```python
from build123d import *

# Parameters (mm, degrees)
SKETCH1_W           = 30
SKETCH1_H           = 44
BOSS_EXTRUDE2_DEPTH = 1


with BuildPart() as part:
    # Sketch1 → Boss-Extrude2 (new body)
    with BuildSketch(Plane.XY):
        Rectangle(SKETCH1_W, SKETCH1_H)
        with BuildLine():
            Line((-7, 8), (7, 8))
            ThreePointArc((7, 8), (7.707106781, 8.292893219), (8, 9))
            Line((8, 9), (8, 12))
            ThreePointArc((8, 12), (7.707106781, 12.707106781), (7, 13))
            Line((7, 13), (-7, 13))
            ThreePointArc((-7, 13), (-7.707106781, 12.707106781), (-8, 12))
            Line((-8, 12), (-8, 9))
            ThreePointArc((-8, 9), (-7.707106781, 8.292893219), (-7, 8))
        make_face(mode=Mode.SUBTRACT)
        with BuildLine():
            Line((-7, -4), (7, -4))
            ThreePointArc((7, -4), (7.707106781, -3.707106781), (8, -3))
            Line((8, -3), (8, 3))
            ThreePointArc((8, 3), (7.707106781, 3.707106781), (7, 4))
            Line((7, 4), (-7, 4))
            ThreePointArc((-7, 4), (-7.707106781, 3.707106781), (-8, 3))
            Line((-8, 3), (-8, -3))
            ThreePointArc((-8, -3), (-7.707106781, -3.707106781), (-7, -4))
        make_face(mode=Mode.SUBTRACT)
        with BuildLine():
            Line((-7, -13), (7, -13))
            ThreePointArc((7, -13), (7.707106781, -12.707106781), (8, -12))
            Line((8, -12), (8, -9))
            ThreePointArc((8, -9), (7.707106781, -8.292893219), (7, -8))
            Line((7, -8), (-7, -8))
            ThreePointArc((-7, -8), (-7.707106781, -8.292893219), (-8, -9))
            Line((-8, -9), (-8, -12))
            ThreePointArc((-8, -12), (-7.707106781, -12.707106781), (-7, -13))
        make_face(mode=Mode.SUBTRACT)
    extrude(amount=BOSS_EXTRUDE2_DEPTH)


solid = part.part
```
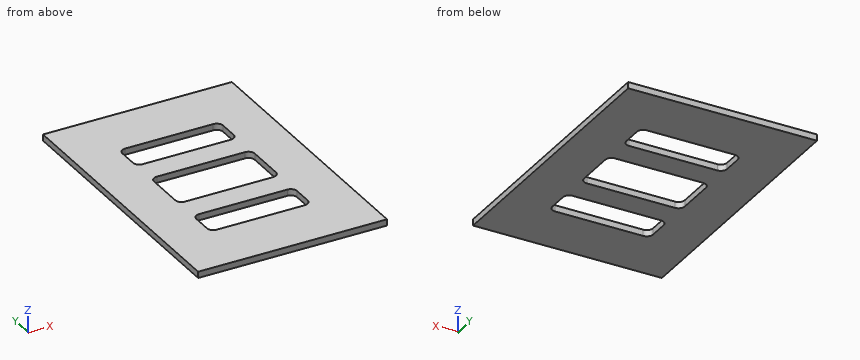
Input: part model. Units: mm. Frame: model coordinates. Coordinates: 2 decimals unless noted, no trailing zeros. Loops run counter-clockwise (first coordinate to the right, second up) from the corner with the lowest first, then second, coordinate; pieces in that order, holes last. Notation, with made-up numbers: M 53,-25 L 82,-25 A27 ccw 82,-7 Z; hole C 19.25,14.25 d8. An arc over 180 degrees is marked long. One line per item, written item: value.
(1) Section A-A (y = 2). Output: boundary loops of the cut face in (x, z).
Filled in:
outline: M -15,0 L -8,0 L -8,1 L -15,1 Z; M 8,0 L 15,0 L 15,1 L 8,1 Z
(2) Section C-C (z = 0.45). Output: boundary loops of the cut face in (x, y).
Filled in:
outline: M -15,-22 L 15,-22 L 15,22 L -15,22 Z; hole M -8,-12 A1 ccw -7,-13 L 7,-13 A1 ccw 8,-12 L 8,-9 A1 ccw 7,-8 L -7,-8 A1 ccw -8,-9 Z; hole M -8,-3 A1 ccw -7,-4 L 7,-4 A1 ccw 8,-3 L 8,3 A1 ccw 7,4 L -7,4 A1 ccw -8,3 Z; hole M -8,9 A1 ccw -7,8 L 7,8 A1 ccw 8,9 L 8,12 A1 ccw 7,13 L -7,13 A1 ccw -8,12 Z
(3) Section B-B (x = -0.25). Output: boundary loops of the cut face in (y, z).
Filled in:
outline: M -22,0 L -13,0 L -13,1 L -22,1 Z; M -8,0 L -4,0 L -4,1 L -8,1 Z; M 4,0 L 8,0 L 8,1 L 4,1 Z; M 13,0 L 22,0 L 22,1 L 13,1 Z
(4) Line query: line 1 along Y through (x, z) = (6.75, 0.6); line 2 along X through (y, z) = (-11, 0.8). Output: solid intervals per line, ascending. Write a range as from..to.
Filled in:
line 1: -22..-13, -8..-4, 4..8, 13..22
line 2: -15..-8, 8..15
